```python
from build123d import *

# Parameters (mm, degrees)
SKETCH_W        = 75
SKETCH_H        = 30
SKETCH_R        = 1.75
SKETCH_W_2      = 15
SKETCH_H_2      = 20
PAD_DEPTH       = 5
FILLET_R        = 10
FILLET001_R     = 1
SKETCH001_W     = 5
SKETCH001_H     = 30
PAD001_DEPTH    = 40
FILLET002_R     = 5
FILLET003_R     = 17
SKETCH002_R     = 2.25
POCKET_DEPTH    = 75.001
CHAMFER_SIZE    = 10
CHAMFER001_SIZE = 0.5


with BuildPart() as part:
    # Sketch → Pad (new body)
    with BuildSketch(Plane.XY):
        with Locations((27.5, 0)):
            Rectangle(SKETCH_W, SKETCH_H)
        Circle(SKETCH_R, mode=Mode.SUBTRACT)
        with Locations((40, 0)):
            Circle(SKETCH_R, mode=Mode.SUBTRACT)
        with Locations((20, 0)):
            Rectangle(SKETCH_W_2, SKETCH_H_2, mode=Mode.SUBTRACT)
    extrude(amount=PAD_DEPTH)

    # Fillet
    fillet_edges = [part.edges().sort_by_distance(p)[0] for p in [
        (-10, 15, 2.5),
        (-10, -15, 2.5),
    ]]
    fillet(fillet_edges, radius=FILLET_R)

    # Fillet001
    fillet001_edges = [part.edges().sort_by_distance(p)[0] for p in [
        (12.5, 0, 5),
        (12.5, 0, 0),
        (20, 10, 0),
        (20, 10, 5),
        (27.5, 0, 5),
        (20, -10, 5),
        (27.5, 0, 0),
        (20, -10, 0),
    ]]
    fillet(fillet001_edges, radius=FILLET001_R)

    # Sketch001 (on Face18 of Fillet001) → Pad001 (join)
    with BuildSketch(Plane.XY.offset(5)):
        with Locations((62.5, 0)):
            Rectangle(SKETCH001_W, SKETCH001_H)
    extrude(amount=PAD001_DEPTH)

    # Fillet002
    fillet002_edges = [part.edges().sort_by_distance(p)[0] for p in [
        (65, 0, 0),
    ]]
    fillet(fillet002_edges, radius=FILLET002_R)

    # Fillet003
    fillet003_edges = [part.edges().sort_by_distance(p)[0] for p in [
        (60, 0, 5),
    ]]
    fillet(fillet003_edges, radius=FILLET003_R)

    # Sketch002 (on Face9 of Fillet003) → Pocket (cut, through all)
    with BuildSketch(Plane.YZ.offset(65)):
        with Locations((0, 39)):
            Circle(SKETCH002_R)
        with Locations((0, 24)):
            Circle(SKETCH002_R)
    extrude(amount=-POCKET_DEPTH, mode=Mode.SUBTRACT)

    # Chamfer
    chamfer_edges = [part.edges().sort_by_distance(p)[0] for p in [
        (62.5, -15, 45),
        (62.5, 15, 45),
    ]]
    chamfer(chamfer_edges, length=CHAMFER_SIZE)

    # Chamfer001
    chamfer001_edges = [part.edges().sort_by_distance(p)[0] for p in [
        (60, -2.25, 39),
        (60, -1.171165, 25.921165),
        (60, 1.921165, 22.828835),
        (38.25, 0, 5),
        (-1.75, 0, 5),
    ]]
    chamfer(chamfer001_edges, length=CHAMFER001_SIZE)


solid = part.part
```
Design review of the part built by this model. Coordinates are the model's own, in mm. A direction names the side the tool comes from. Give positions to 0.01 mm unless a question says otherwise; leave off trailing zeros. Write each loop counter-clockwise with the first axis right and the second up, starting at its lowest first coordinate (ties: lowest second). Pieces come first, ordered by that corner, then holes. Notation, with made-up numbers: (52, 19) - (58, 19) arc R25 cw to (58, 53) - close; hole circle Ø3 at (-27, -17). An arc over 180 degrees is marked (long way). Return JSON: item names as keys, results as strings. Group by question number.
(1) Insertion check: pin 1 (6 mm diameter, centred on x = 11, y = -3.5, fed in from +Z); pin 2 (0.9 mm diameter, centred on y = -0.5, z = 2, fed in from +X); pin 3 (4 mm diameter, centred on x = 40, y = 0, fed in from +Z). Each pin has a flat end and moves straight along its axis. Give the tip position at first contact, or say it passes through.
(2) Machinability: for faces 1 (the flat face through (65, 0, 20)), 2 (the flat face through (10, 0, 5)), 3 (the flat face through (27.5, 0, 2)), which of the approach directions +Z, -Z, +X, -X, +Y, -Y give a long, thin tool a straight path to every point of the face, cutting with its end or side? Answer none if there is none.
(3) We need section B-B, the plane z = 24. Give the boundary of the cut face in (x, y), then the cut area to 3 significant figures.
(4) We need section A-A, the plane x = 23. Give the boundary of the cut face in (y, z), then the cut area to 3 significant figures.
(5) We need section C-C, the plane x = 40. Give the boundary of the cut face in (y, z), then the cut area to 3 significant figures.
(6) Mouldability with a two-part tool opening along Y and no side actions: class faces 4 (the cylindrical face through (1.617, -0.67, 2.218)), 5 (the flat face through (20, 10, 2)), 6 (the flat face through (-10, 0, 2)), 7 (the flat face through (62, -10, 40)) as +Y half, -Y half, draft (parallel to the pull), parting line (faces both ways), or undercut.
(7) To check wall thickness, follow probe 1 along Y at (x, z) = (40, 1.5); probe 2 along Y at (x, z) = (63.35, 24); probe 3 along X at (y, z) = (4, 34). State the ranges of each line that lie inside material, in increasing order.
(8) We need section D-D, the plane z = 3. Give the boundary of the cut face in (x, y).
Reported:
{
 "1": {"pin 1": "stops at z = 5", "pin 2": "stops at x = 64.3", "pin 3": "stops at z = 4.75"},
 "2": {"face 1": "+Z, -Z, +X, +Y, -Y", "face 2": "+Z, -X, +Y, -Y", "face 3": "+Z, -Z"},
 "3": {"outline": "(60, -15) - (65, -15) - (65, -2.25) - (60.5, -2.25) - (60, -2.75) - close; (60, 2.75) - (60.5, 2.25) - (65, 2.25) - (65, 15) - (60, 15) - close", "area": "127 mm2"},
 "4": {"outline": "(-15, 0) - (-11, 0) arc R1 ccw to (-10, 1) - (-10, 4) arc R1 ccw to (-11, 5) - (-15, 5) - close; (10, 1) arc R1 ccw to (11, 0) - (15, 0) - (15, 5) - (11, 5) arc R1 ccw to (10, 4) - close", "area": "49.1 mm2"},
 "5": {"outline": "(-15, 0) - (-1.75, 0) - (-1.75, 4.5) - (-2.25, 5) - (-15, 5) - close; (1.75, 0) - (15, 0) - (15, 5) - (2.25, 5) - (1.75, 4.5) - close", "area": "132 mm2"},
 "6": {"face 4": "undercut", "face 5": "undercut", "face 6": "draft", "face 7": "-Y half"},
 "7": {"probe 1": "y = -15 to -1.75, 1.75 to 15", "probe 2": "y = -15 to -2.25, 2.25 to 15", "probe 3": "x = 60 to 65"},
 "8": {"outline": "(-10, -5) arc R10 ccw to (0, -15) - (64.58, -15) - (64.58, 15) - (0, 15) arc R10 ccw to (-10, 5) - close; hole circle Ø3.5 at (0, 0); hole (12.5, -10) - (27.5, -10) - (27.5, 10) - (12.5, 10) - close; hole circle Ø3.5 at (40, 0)"}
}
